Design review of the part shown in the three views and the two pictorial views. Dimensions are in mm from the part's minimum x, y and z. A direction names the side the tool comes from. Round coordinates to 2 decimals unless told otherwise and drop trailing zeros. Loops run counter-clockwise (first coordinate to the right, second up) from the corner with the lowest first, then second, coordinate; pieces in that order, holes last.
1) Take a section at A-A (z = 36). State the section outline as (x, y) points.
2) Wall thickness on L1, parallel to Z at x = 95, y = 17.5; L2, parallel to Y at x = 89.5, z = 18 (1 decimal); L3, parallel to X at y = 4, z = 9: over which ranges is each line inside the solid? List them lowest first.
3) Take a section at D-D (z = 11). State the section outline as (x, y) points.
4) Insertion check: pin 1 (9 mm diameter, centred on x = 85.22, y = 58.33, fed in from -Z); pin 2 (4 mm diameter, centred on x = 22, z = 63, fed in from -Y); pin 3 (4 mm diameter, centred on y = 55.5, z = 66, fed in from +X); pin 4 (6 mm diameter, centred on y = 9, z = 35, fed in from -X). Each pin has a flat end and moves straight along its axis. Give the tip position at first contact, or say it passes through.
5) Tool access review of the marked faces 1 and 2: name each direction out of +Z, -Z, +X, -X, +Y, -Y from which nothing blocks a thin tool from reaching the whole face with its end or side.
6) Mouldability with a two-part tool opening along Y and no side actions: class the marked faces 3, 4, 5 and 6 as pulls with the +Y half, pulls with the -Y half, needs draft (parallel to the pull), parting line crosses it, or undercut.
7) Take a section at C-C (x = 16). State the section outline as (y, z) points.
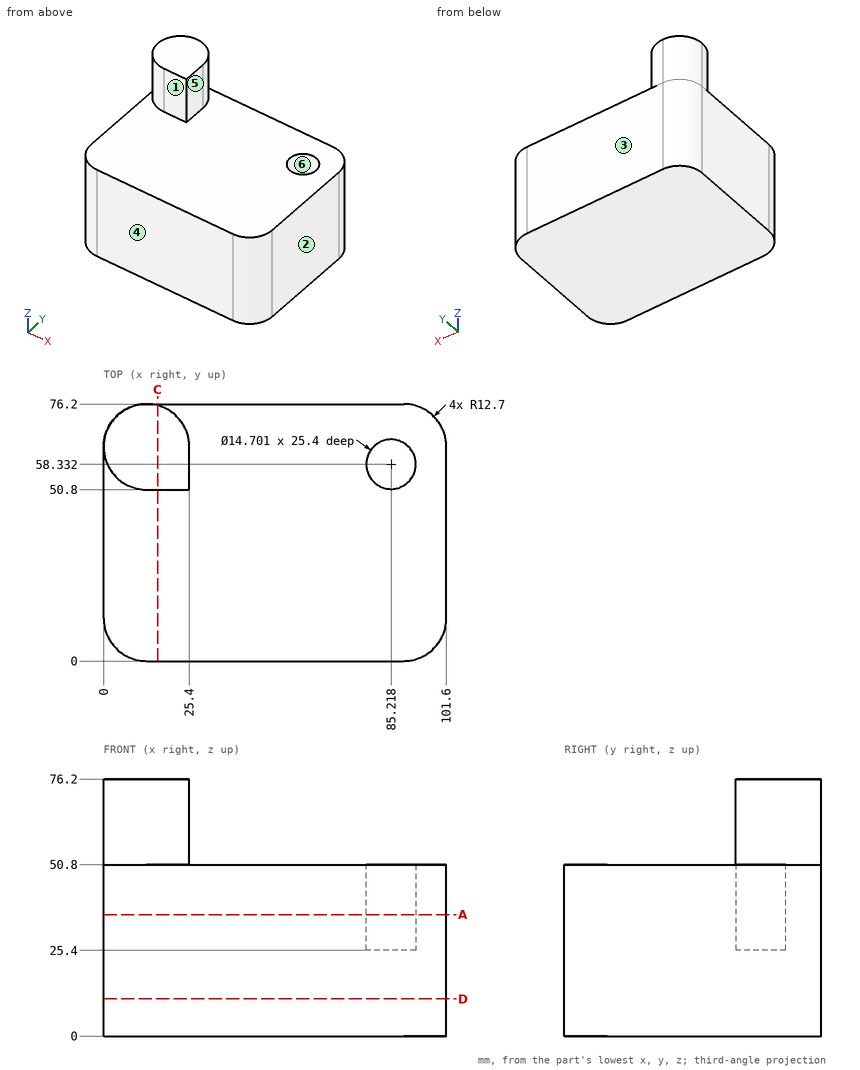
Response:
1. outline: (0, 12.7) arc R12.7 ccw to (12.7, 0) - (88.9, 0) arc R12.7 ccw to (101.6, 12.7) - (101.6, 63.5) arc R12.7 ccw to (88.9, 76.2) - (12.7, 76.2) arc R12.7 ccw to (0, 63.5) - close; hole circle Ø14.7 at (85.22, 58.33)
2. L1: z = 0 to 50.8
2. L2: y = 0 to 76.2
2. L3: x = 3.45 to 98.15
3. outline: (0, 12.7) arc R12.7 ccw to (12.7, 0) - (88.9, 0) arc R12.7 ccw to (101.6, 12.7) - (101.6, 63.5) arc R12.7 ccw to (88.9, 76.2) - (12.7, 76.2) arc R12.7 ccw to (0, 63.5) - close
4. pin 1: stops at z = 0
4. pin 2: stops at y = 50.8
4. pin 3: stops at x = 25.4
4. pin 4: stops at x = 0.02
5. face 1: +Z, +X, -X, -Y
5. face 2: +Z, -Z, +X, +Y, -Y
6. face 3: pulls with the +Y half
6. face 4: pulls with the -Y half
6. face 5: needs draft
6. face 6: undercut
7. outline: (0, 0) - (76.2, 0) - (76.2, 50.8) - (75.76, 50.8) - (75.76, 76.2) - (50.8, 76.2) - (50.8, 50.8) - (0, 50.8) - close
